For this review, take the finished solid that the model builds, in its own axes (mm). Face numbers are marked on the shaded views. A direction names the side the tool comes from. Round coordinates to 2 decimals unless told otherwise and drop trailing zeros. Write each loop counter-clockwise with the first axis right and the second up, starting at its lowest first coordinate (ties: lowest second). Pieces come first, ordered by that corner, then holes. Notation, with made-up numbers: M -5.75,20.25 L 47.25,20.25 A29 ccw 47.25,56.25 Z; hole C 69.5,38 d3. An arc over 180 degrees is marked long. Use one line per item in the form item = value. Start each with the question number.
Item 1: For P1, Ø4, axis at x = -74, y = -69.85, coming from the +Z side; P2, Ø1.5, axis at y = -70.5, z = -34.5, coming from the +X side; P3, Ø6.5, axis at y = -70, z = -33.5, coming from the -X side; P4, Ø3, axis at x = -75.5, y = -72.5, coming from the +Z side, all flat-tipped, find the tip position at first contact; note any pin that passes through.
Item 2: Add section B-B (z = -29). State the section outline as (x, y) points.
Item 3: For the marked faces 1, 2 and 3, list the 3-axis set-ups (+Z, -Z, +X, -X, +Y, -Y) from which the entire face can be reached by the end or side of a thin tool; tool diameter is ignored.
Item 4: Draft analysis for pull direction Z (two halves, no side actions). For the marked faces 4, 5 and 6, state which applies: released by +Z, released by -Z, zero draft, split by the parting line, or undercut.
Item 5: Add section C-C (x = -79). State the section outline as (y, z) points.
Item 6: Add section D-D (z = -34.75). State the section outline as (x, y) points.
Item 7: For line 1 (Y direction, x = -84, z = -33.75); line 2 (Y direction, x = -74, z = -30.25); line 3 (Z direction, x = -72, y = -71), list the stretches that pass through material, from the lowest coordinate up. Write a range as [from, to].
Item 8: Add section A-A (y = -70). State the section outline as (x, z) points, and give its area (3 significant figures).
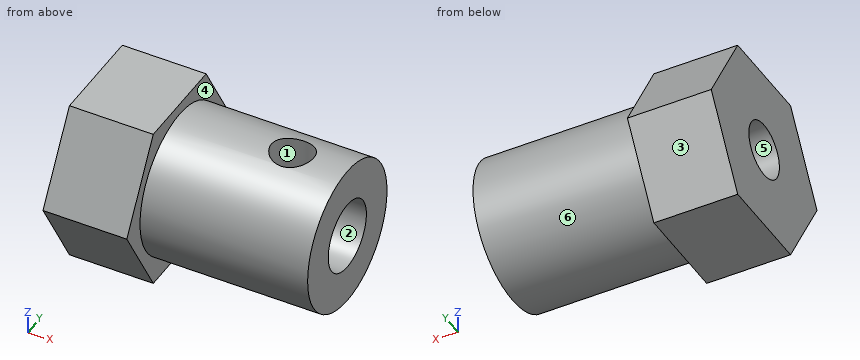
from build123d import *

# Parameters (mm, degrees)
EXTRUDE_1_DEPTH                = 6
SKETCH_2_W                     = 12
SKETCH_2_H                     = 5.2
HOLE_WIZARD_M3_5_1_D           = 4
HOLE_WIZARD_M3_5_1_CBORE_D     = 5
HOLE_WIZARD_M3_5_1_CBORE_DEPTH = 12
SKETCH_5_W                     = 1.5
SKETCH_5_H                     = 4.122312264


with BuildPart() as part:
    # 草图1 → 凸台-拉伸1 (new body)
    with BuildSketch(Plane(origin=(-88, 0, 0), x_dir=(0, -1, 0), z_dir=(-1, 0, 0))):
        Polygon((76.92820323, -33.5), (73.464101615, -27.5), (66.535898385, -27.5), (63.07179677, -33.5), (66.535898385, -39.5), (73.464101615, -39.5), align=None)
    extrude(amount=-EXTRUDE_1_DEPTH)

    # 草图2 → 旋转1 (revolve)
    with BuildSketch(Plane(origin=(0, 0, -33.5), x_dir=(-1, 0, 0), z_dir=(0, 0, -1)), mode=Mode.PRIVATE) as revolve_1_sk:
        with Locations((76, -67.4)):
            Rectangle(SKETCH_2_W, SKETCH_2_H)
    revolve(revolve_1_sk.sketch.rotate(Axis((-70, -70, -33.5), (-1, 0, 0)), 270), axis=Axis((-70, -70, -33.5), (-1, 0, 0)))

    # M3.5 六角头机械螺钉的柱形沉头孔1 (through all)
    with Locations(Plane(origin=(-70, 0, 0), x_dir=(0, 0, -1), z_dir=(1, 0, 0))):
        with Locations((33.5, -70)):
            CounterBoreHole(HOLE_WIZARD_M3_5_1_D / 2, HOLE_WIZARD_M3_5_1_CBORE_D / 2, HOLE_WIZARD_M3_5_1_CBORE_DEPTH)

    # 草图5 → Ø3.0 (3) 直径孔1 (revolve, cut)
    with BuildSketch(Plane(origin=(-74, -69.849458039, -31.622312264), x_dir=(0, 1, 0), z_dir=(1, 0, 0))):
        with Locations((0.75, 2.061156132)):
            Rectangle(SKETCH_5_W, SKETCH_5_H)
    revolve(axis=Axis((-74, -69.849458039, -37.972312264), (0, 0, 1)), mode=Mode.SUBTRACT)


solid = part.part
Calculated:
q1.P1 = -28.3
q1.P2 = through
q1.P3 = -88
q1.P4 = -28.4
q2.outline = M -88,-74.33 L -82,-74.33 L -82,-72.61 L -70,-72.61 L -70,-67.39 L -82,-67.39 L -82,-65.67 L -88,-65.67 Z; hole C -74,-69.85 d3
q3.face_1 = +Z
q3.face_2 = +X
q3.face_3 = -Z, +X, -X, +Y
q4.face_4 = zero draft
q4.face_5 = undercut
q4.face_6 = split by the parting line
q5.outline = C -70,-33.5 d10.4; hole C -70,-33.5 d5
q6.outline = M -88,-76.21 L -82,-76.21 L -82,-75.05 L -70,-75.05 L -70,-72.17 L -82,-72.17 L -82,-71.56 L -88,-71.56 Z; M -88,-68.44 L -82,-68.44 L -82,-67.83 L -70,-67.83 L -70,-64.95 L -82,-64.95 L -82,-63.79 L -88,-63.79 Z
q7.line_1 = [-76.78, -71.98], [-68.02, -63.22]
q7.line_2 = [-74.06, -71.35], [-68.35, -65.94]
q7.line_3 = [-38.6, -35.79], [-31.21, -28.4]
q8.outline = M -88,-39.5 L -82,-39.5 L -82,-38.7 L -70,-38.7 L -70,-36 L -82,-36 L -82,-35.5 L -88,-35.5 Z; M -88,-31.5 L -82,-31.5 L -82,-31 L -75.49,-31 L -75.49,-28.3 L -82,-28.3 L -82,-27.5 L -88,-27.5 Z; M -72.51,-31 L -70,-31 L -70,-28.3 L -72.51,-28.3 Z
q8.area = 105 mm^2
